Drawing for the job (mm, zero at the part's lowest x, y, z). A direction names the side the tool comes from. Coordinates: 2 decimals unless noted, no trailing zeros. Order: outer loops, then holes, each group sorted by start corner. A loop starts at its lowest first (then second) coordinate and runs counter-clockwise, first axis right, second up.
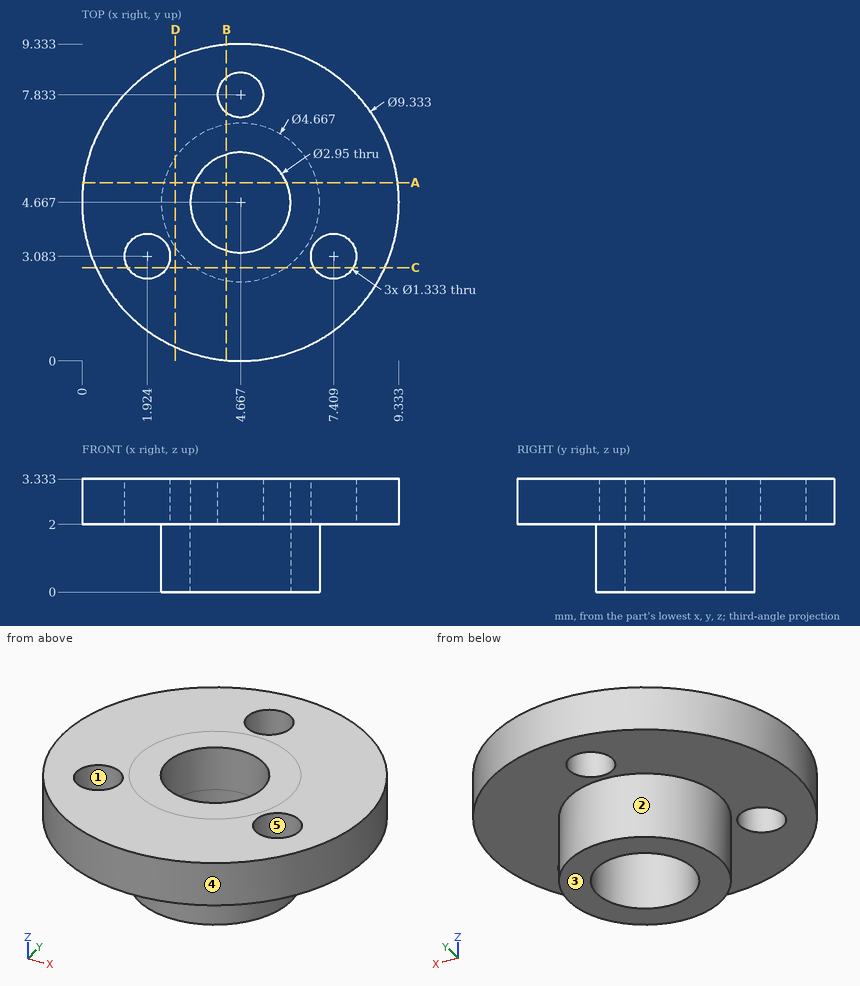
(1) Probe line 1 (X direction, y = 4.75, z = 1.45) (1 decimal); line 2 (Z direction, x = 1.5, y = 6.75). List the from-to ranges inside material, lowest first.
(2) Drop a flat-ended pin along its axis: pin 1 (0.8 mm diameter, centred on x = 4.67, y = 7.83, fed in from -Z). Give the stop position or say it passes through.
(3) Slice it at D-D, the plane x = 2.75. Give the cut face in (y, z), then the cut area to 3 significant figures.
(4) Slice it at B-B, the plane x = 4.25. State how many separate pieces and enclosed holes the cut face has.
(5) Slice it at C-C, the plane y = 2.75. Give the cut face in (x, z).
(6) Tool access for the marked faces 1 and 2: list every direction of +Z, -Z, +X, -X, +Y, -Y with a clear straight run to the whole face (end or side of a thin tool).
(7) Pull direction Y, two halves, no side cores. Call the marked faces 3, 4 and 5: +Y half, -Y half, draft (parallel to the pull), parting line (faces both ways), or undercut.
(8) Slice it at A-A, the plane y = 5.25. Give the cut face in (x, z).
Here are the results:
1. line 1: x = 2.3 to 3.2, 6.1 to 7
1. line 2: z = 2 to 3.33
2. pin 1: passes through
3. outline: (0.41, 2) - (3.34, 2) - (3.34, 0) - (6, 0) - (6, 2) - (8.92, 2) - (8.92, 3.33) - (0.41, 3.33) - close
3. area: 16.7 mm2
4. separate pieces: 3
4. enclosed holes: 0
5. outline: (0.41, 2) - (1.35, 2) - (1.35, 3.33) - (0.41, 3.33) - close; (2.5, 2) - (3.34, 2) - (3.34, 0) - (6, 0) - (6, 2) - (6.83, 2) - (6.83, 3.33) - (2.5, 3.33) - close; (7.99, 2) - (8.92, 2) - (8.92, 3.33) - (7.99, 3.33) - close
6. face 1: +Z, -Z
6. face 2: -Z
7. face 3: draft
7. face 4: parting line
7. face 5: undercut
8. outline: (0.04, 2) - (2.41, 2) - (2.41, 0) - (3.31, 0) - (3.31, 3.33) - (0.04, 3.33) - close; (6.02, 0) - (6.93, 0) - (6.93, 2) - (9.3, 2) - (9.3, 3.33) - (6.02, 3.33) - close
